Part model, mm, in its own coordinate system. Give positions to 0.01 mm unless a question says otherwise; leave off trailing zeros. Write each loop counter-clockwise with the first axis right and the second up, starting at its lowest first coordinate (ties: lowest second). Pieces come first, ordered by that corner, then holes.
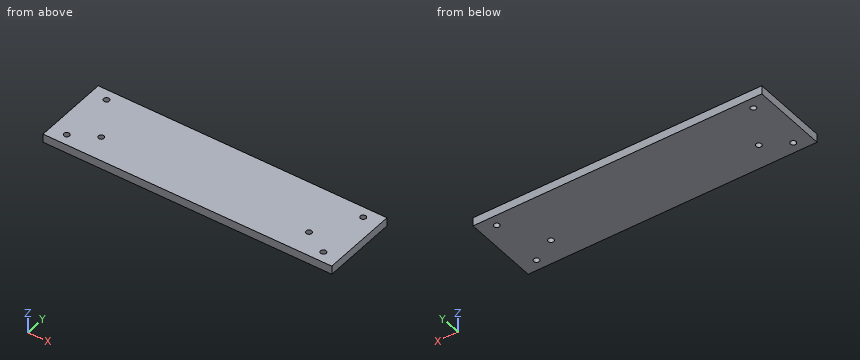
Autodesk Inventor part; units mm, degrees
ref_plane "YZ Plane" through (0, 0, 0) normal (1, 0, 0) x (0, 1, 0)
ref_plane "XZ Plane" through (0, 0, 0) normal (0, 1, 0) x (-1, 0, 0)
ref_plane "XY Plane" through (0, 0, 0) normal (0, 0, 1) x (1, 0, 0)
sketch "Sketch1" plane through (0, 0, 0) normal (0, 0, 1) x (1, 0, 0)
  line L0 (0, 0) -> (215.9, 0)
  line L1 (215.9, 0) -> (215.9, 57.15)
  line L2 (215.9, 57.15) -> (0, 57.15)
  line L3 (0, 57.15) -> (0, 0)
  dimension "d0" = 215.9
  dimension "d1" = 57.15
extrude "Extrusion1" add sketch "Sketch1" along normal blind 6.35
sketch "Sketch2" plane through (0, 0, 6.35) normal (0, 0, 1) x (1, 0, 0)
  line L0 (0, 57.15) -> (0, 0)
  line L1 (0, 57.15) -> (0, 49.15)
  line L2 (0, 49.15) -> (12, 49.15)
  circle A0 centre (12, 49.15) radius 2.1
  line L3 (0, 0) -> (0, 8)
  line L4 (0, 8) -> (12, 8)
  circle A1 centre (12, 8) radius 2.1
  line L5 (215.9, 0) -> (215.9, 57.15)
  line L6 (215.9, 57.15) -> (215.9, 49.15)
  line L7 (215.9, 49.15) -> (203.9, 49.15)
  circle A2 centre (203.9, 49.15) radius 2.1
  line L8 (215.9, 0) -> (215.9, 8)
  line L9 (215.9, 8) -> (203.9, 8)
  circle A3 centre (203.9, 8) radius 2.1
  dimension "d4" = 8
  dimension "d5" = 12
  dimension "d6" = 4.2
  dimension "d7" = 8
  dimension "d8" = 12
  dimension "d9" = 4.2
  dimension "d10" = 12
  dimension "d11" = 4.2
  dimension "d12" = 12
  dimension "d13" = 4.2
extrude "Extrusion2" cut sketch "Sketch2" against normal through all
sketch "Sketch3" plane through (0, 0, 6.35) normal (0, 0, 1) x (1, 0, 0)
  line L0 (0, 0) -> (30.25, 0)
  line L1 (0, 0) -> (215.9, 0)
  line L2 (30.25, 0) -> (30.25, 18.35)
  circle A0 centre (30.25, 18.35) radius 2.1
  line L3 (215.9, 0) -> (185.65, 0)
  line L4 (185.65, 0) -> (185.65, 18.35)
  circle A1 centre (185.65, 18.35) radius 2.1
  dimension "d16" = 30.25
  dimension "d17" = 18.35
  dimension "d18" = 4.2
  dimension "d19" = 30.25
  dimension "d20" = 18.35
  dimension "d21" = 4.2
extrude "Extrusion3" cut sketch "Sketch3" against normal blind 25.4
properties part number "SideRail"
1) Drill centre lines: L1, parallel to Y at x = 203.9, z = 4; L2, parallel to X at y = 18.35, z = 5; L3, parallel to Y at x = 30.25, z = 5. Where is each one in solid material? Low to high.
Check result:
L1: y = 0 to 5.9, 10.1 to 47.05, 51.25 to 57.15
L2: x = 0 to 28.15, 32.35 to 183.55, 187.75 to 215.9
L3: y = 0 to 16.25, 20.45 to 57.15
2) Saw through at A-A (y = 49.15). Write the cut outline in (x, z).
Check result:
outline: (0, 0) - (9.9, 0) - (9.9, 6.35) - (0, 6.35) - close; (14.1, 0) - (201.8, 0) - (201.8, 6.35) - (14.1, 6.35) - close; (206, 0) - (215.9, 0) - (215.9, 6.35) - (206, 6.35) - close
3) Flat gauge pins, fed straight in: P1, Ø3.5, axis at x = 12, y = 49.15, coming from the +Z side; P2, Ø12, axis at x = 120.5, y = 42, coming from the -Z side. Where does each tip first touch, or does it go through?
Check result:
P1: passes through
P2: stops at z = 0
4) Saw through at B-B (x = 203.9). Write the cut outline in (y, z), and give its area (3 significant figures).
Check result:
outline: (0, 0) - (5.9, 0) - (5.9, 6.35) - (0, 6.35) - close; (10.1, 0) - (47.05, 0) - (47.05, 6.35) - (10.1, 6.35) - close; (51.25, 0) - (57.15, 0) - (57.15, 6.35) - (51.25, 6.35) - close
area: 310 mm2
